from build123d import *

# Parameters (mm, degrees)
ESQUISSE1_R                  = 25
BOSS_EXTRU_1_DEPTH           = 51.2
ESQUISSE2_R                  = 20
BOSS_EXTRU_2_DEPTH           = 18.8
ESQUISSE3_R                  = 16.5
BOSS_EXTRU_3_DEPTH           = 16.7
ESQUISSE4_R                  = 27.5
BOSS_EXTRU_4_DEPTH           = 47.1
CHANFREIN1_SIZE              = 10
CHANFREIN1_SIZE2             = 17.320508076
ESQUISSE12_R                 = 6.35
ENL_V_MAT_EXTRU_1_DEPTH      = 28.5
ENL_V_MAT_EXTRU_1_DEPTH_BACK = 28.5
ESQUISSE13_R                 = 47.258439022
ENL_V_MAT_EXTRU_2_DEPTH      = 15
ESQUISSE14_R                 = 39.934727028
ESQUISSE14_R_2               = 7.5
ENL_V_MAT_EXTRU_4_DEPTH      = 32.5


with BuildPart() as part:
    # Esquisse1 → Boss.-Extru.1 (new body)
    with BuildSketch(Plane.XY):
        Circle(ESQUISSE1_R)
    extrude(amount=BOSS_EXTRU_1_DEPTH)

    # Esquisse2 → Boss.-Extru.2 (add)
    with BuildSketch(Plane.XY.offset(51.2)):
        Circle(ESQUISSE2_R)
    extrude(amount=BOSS_EXTRU_2_DEPTH)

    # Esquisse3 → Boss.-Extru.3 (add)
    with BuildSketch(Plane.XY.offset(70)):
        Circle(ESQUISSE3_R)
    extrude(amount=BOSS_EXTRU_3_DEPTH)

    # Esquisse4 → Boss.-Extru.4 (add)
    with BuildSketch(Plane.XY.offset(86.7)):
        Circle(ESQUISSE4_R)
    extrude(amount=BOSS_EXTRU_4_DEPTH)

    # Chanfrein1
    chanfrein1_edges = [part.edges().sort_by_distance(p)[0] for p in [
        (-27.5, 0, 86.7),
    ]]
    chanfrein1_side = [part.faces().sort_by_distance(p)[0] for p in [
        (-26.722182541, 0, 86.7),
    ]]
    chamfer(chanfrein1_edges, length=CHANFREIN1_SIZE, length2=CHANFREIN1_SIZE2, reference=chanfrein1_side[0])

    # Esquisse12 → Enlèv. mat.-Extru.1 (cut, two sides)
    with BuildSketch(Plane(origin=(0, 0, 0), x_dir=(1, 0, 0), z_dir=(0, 1, 0))) as enl_v_mat_extru_1_sk:
        with Locations((0, -15)):
            Circle(ESQUISSE12_R)
    extrude(amount=ENL_V_MAT_EXTRU_1_DEPTH, mode=Mode.SUBTRACT)
    extrude(enl_v_mat_extru_1_sk.sketch, amount=-ENL_V_MAT_EXTRU_1_DEPTH_BACK, mode=Mode.SUBTRACT)

    # Esquisse13 → Enlèv. mat.-Extru.2 (cut)
    with BuildSketch(Plane.XY.offset(133.8)):
        with Locations((0.544033406, 0)):
            Circle(ESQUISSE13_R)
    extrude(amount=-ENL_V_MAT_EXTRU_2_DEPTH, mode=Mode.SUBTRACT)

    # Esquisse14 → Enlèv. mat.-Extru.4 (cut)
    with BuildSketch(Plane.XY.offset(118.8)):
        Circle(ESQUISSE14_R)
        Circle(ESQUISSE14_R_2, mode=Mode.SUBTRACT)
    extrude(amount=-ENL_V_MAT_EXTRU_4_DEPTH, mode=Mode.SUBTRACT)


solid = part.part
Input: part model. Units: mm. Frame: model coordinates. A direction names the side the tool comes from. Coordinates: 2 decimals unless noted, no trailing zeros. Order: outer loops, then holes, each group sorted by start corner. A loop starts at its lowest first (then second) coordinate and runs counter-clockwise, first axis right, second up. Notation, with made-up numbers: M -2.75,29.5 L 32.25,29.5 A10 cw 32.25,48.5 Z; hole C 73.25,12.5 d3. An arc over 180 degrees is marked long. Answer as CSV lines item,"result".
1. Access query for faces 4 (the cylindrical face through (-4.336, -19.524, 60.468)), 5 (the flat face through (0, 0, 0)). Directions: +Z, -Z, +X, -X, +Y, -Y. A direction counts if a zero-diameter tool reaches every point of the face in a straight line with its end or side. Return the directions, or none.
Reported:
face 4,"+Z"
face 5,"-Z, +X, -X, +Y, -Y"
2. Section C-C (y = 13). Return the cut outline in (x, z), then the cut area to 3 significant figures.
Reported:
outline,"M -21.35,0 L 21.35,0 L 21.35,51.2 L 15.2,51.2 L 15.2,70 L 10.16,70 L 10.16,86.3 L -10.16,86.3 L -10.16,70 L -15.2,70 L -15.2,51.2 L -21.35,51.2 Z; hole C 0,15 d12.7"
area,"2,960 mm2"
3. Section A-A (y = 0). Return the cut outline in (x, z), then the cut area to 3 significant figures.
Reported:
outline,"M -25,0 L 25,0 L 25,51.2 L 20,51.2 L 20,70 L 16.5,70 L 16.5,86.3 L 7.5,86.3 L 7.5,118.8 L -7.5,118.8 L -7.5,86.3 L -16.5,86.3 L -16.5,70 L -20,70 L -20,51.2 L -25,51.2 Z; hole C 0,15 d12.7"
area,"4,210 mm2"
4. Pull-direction query (X, two-part tool) for faces 1 (the flat face through (2.9, 16.4, 70)), 2 (the cylindrical face through (-7.493, 0.33, 102.778)), 3 (the cylindrical face through (2.93, 0.35, 20.634)); classes: released by +X, released by -X, zero draft, split by the parting line, or undercut.
Reported:
face 1,"zero draft"
face 2,"split by the parting line"
face 3,"undercut"
5. First-contact query: P1, Ø16.5, axis at x = 0, z = 15, coming from the +Y side; P2, Ø12, axis at x = -16.5, z = 42.5, coming from the +Y side; P3, Ø15, axis at x = -10, y = -12.5, coming from the +Z side; P4, Ø1.5, axis at x = 14, y = -13, coming from the +Z side. Flat tips, straight axial feed; report the tip coordinate or a pass-through.
Reported:
P1,"y = 25"
P2,"y = 22.69"
P3,"z = 86.3"
P4,"z = 70"
6. Section B-B (x = 0). Return the cut outline in (y, z).
Reported:
outline,"M -25,0 L 25,0 L 25,8.65 L -25,8.65 Z; M -25,21.35 L 25,21.35 L 25,51.2 L 20,51.2 L 20,70 L 16.5,70 L 16.5,86.3 L 7.5,86.3 L 7.5,118.8 L -7.5,118.8 L -7.5,86.3 L -16.5,86.3 L -16.5,70 L -20,70 L -20,51.2 L -25,51.2 Z"
7. Material intervals for line 1 (Z direction, x = 0, y = 6); line 2 (Z direction, x = 21.5, y = -9); line 3 (Z direction, x = -7, y = -13), sorted ascending. Write a range as from..to.
Reported:
line 1,"0..8.65, 21.35..118.8"
line 2,"0..51.2"
line 3,"0..86.3"
8. Section D-D (z = 58.5). Return the cut outline in (x, y), then the cut area to 3 significant figures.
Reported:
outline,"C 0,0 d40"
area,"1,260 mm2"
